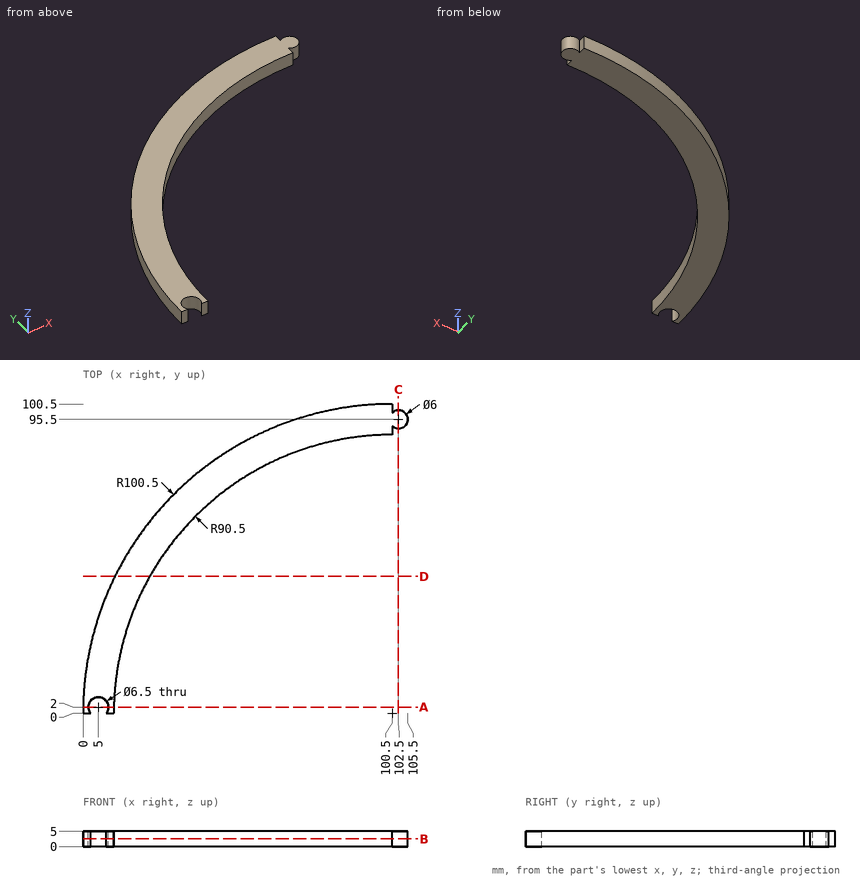
Part print with two shaded views. Sizes in mm from the minimum x, y, z corner. Round coordinates to 2 decimals unless told otherwise and drop trailing zeros. Loops run counter-clockwise (first coordinate to the right, second up) from the corner with the lowest first, then second, coordinate; pieces in that order, holes last. Notation, with made-up numbers: M -1.5,16 L 44.5,16 A25 cw 44.5,43 Z; hole C 27.5,-4 d7. An arc over 180 degrees is marked long. Return JSON: item names as keys, results as strings. Group by question number.
(1) Saw through at A-A, the plane y = 2. List the corners of the cut face in (x, z).
(2) Wall check: probe 1 along X at (y, z) = (2, 3.55); probe 2 along X at (y, z) = (7, 3.65); probe 3 along X at (y, z) = (68.5, 3). Give the ranges that are in metal, low to high. Write a range as [from, to].
(3) Saw through at C-C, the plane x = 102.5. List the corners of the cut face in (y, z).
(4) Drop a flat-ended pin along its axis: P1, Ø1.5, axis at y = 80.5, z = 2, coming from the -X side. Give the stop position or say it passes through.
(5) Saw through at D-D, the plane y = 44.5. List the corners of the cut face in (x, z).
(6) Saw through at B-B, the plane z = 2.55. List the corners of the cut face in (x, y).
Answer list:
{
 "1": {"outline": "M 0.02,0 L 1.75,0 L 1.75,5 L 0.02,5 Z; M 8.25,0 L 10.02,0 L 10.02,5 L 8.25,5 Z"},
 "2": {"probe 1": "[0.02, 1.75], [8.25, 10.02]", "probe 2": "[0.24, 10.27]", "probe 3": "[26.96, 41.36]"},
 "3": {"outline": "M 92.5,0 L 98.5,0 L 98.5,5 L 92.5,5 Z"},
 "4": {"P1": "x = 39.34"},
 "5": {"outline": "M 10.39,0 L 21.7,0 L 21.7,5 L 10.39,5 Z"},
 "6": {"outline": "M 0,0 L 2.44,0 A3.25 cw long 7.56,0 L 10,0 A90.5 cw 100.5,90.5 L 100.5,93.26 A3 ccw long 100.5,97.74 L 100.5,100.5 A100.5 ccw Z"}
}
